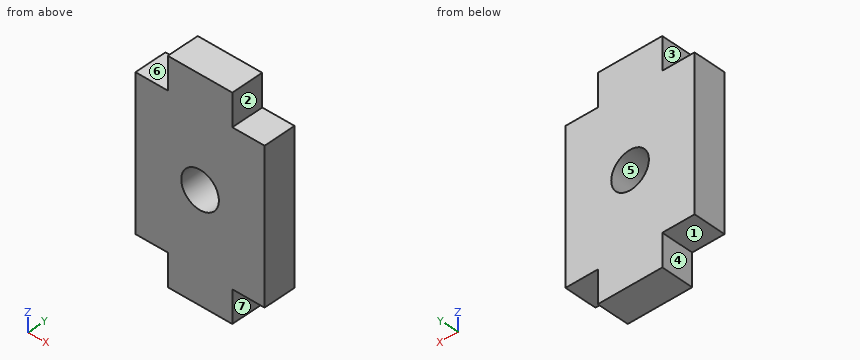
from build123d import *

# Parameters (mm, degrees)
F0_R     = 1.75
F0_W     = 6
F0_H     = 3
F1_DEPTH = 3


with BuildPart() as f1:
    # F0 (on Front) → F1 (new body)
    with BuildSketch(Plane.XZ):
        Polygon((6, -7), (6, 7), (3, 7), (-3, 7), (-6, 7), (-6, -7), (-3, -7), (3, -7), align=None)
        Circle(F0_R, mode=Mode.SUBTRACT)
        with Locations((0, 8.5)):
            Rectangle(F0_W, F0_H)
        with Locations((0, -8.5)):
            Rectangle(F0_W, F0_H)
    extrude(amount=F1_DEPTH)


solid = f1.part
Source: CAD feature listing. Evaluate the final solid. Frame: model axes, mm. Face numbers are marked on the shaded views. A direction names the side the tool comes from. Give positions to 0.01 mm unless a question says otherwise; leave off trailing zeros. Order: outer loops, then holes, each group sorted by start corner. A loop starts at its lowest first (then second) coordinate and runs counter-clockwise, first axis right, second up. Notation, with made-up numbers: (-35.75, 7.5) -> (13.25, 7.5) arc R13 cw to (13.25, 27.5) -> close; hole circle Ø2 at (25.5, 8.5). An arc over 180 degrees is marked (long way). Write item = value, one per line.
Q1. Pin query (flat end, axial travel): pin 1 (0.9 mm diameter, centred on y = -1, z = -8.5, fed in from +X); pin 2 (1.5 mm diameter, centred on x = 4.5, y = -2, fed in from +Z); pin 3 (6 mm diameter, centred on x = -2, z = -1, fed in from +Y); pin 4 (0.9 mm diameter, centred on x = 4, y = -1, fed in from -Z). Return the tip coordinate at first contact, or that it passes through.
Data:
pin_1 = 3
pin_2 = 7
pin_3 = 0
pin_4 = -7
Q2. Set-up query: the marked faces 1, 2 and 3. Return all of +Z, -Z, +X, -X, +Y, -Y with unobstructed straight access to the full face (end or side cutting, diameter ignored); none if empty.
Data:
face_1 = -Z, -X, +Y, -Y
face_2 = +Z, +X, +Y, -Y
face_3 = +Z, -X, +Y, -Y
Q3. Material intervals for line 1 (Z direction, x = 0, y = -1.95); line 2 (Z direction, x = 4.75, y = -1.5); line 3 (X direction, y = -0.55, z = -7.25), sorted ascending. Write a range as from..to.
Data:
line_1 = -10..-1.75, 1.75..10
line_2 = -7..7
line_3 = -3..3
Q4. Pull-direction query (X, two-part tool) for the marked faces 4, 5, 6 and 7; classes: released by +X, released by -X, zero draft, split by the parting line, or undercut.
Data:
face_4 = released by -X
face_5 = undercut
face_6 = zero draft
face_7 = released by +X
Q5. Cut plane D-D, the plane z = 8.75. Output: boundary loops of the cut face in (x, y).
Data:
outline = (-3, -3) -> (3, -3) -> (3, 0) -> (-3, 0) -> close
Q6. Cut plane C-C, the plane y = -1.25. Output: boundary loops of the cut face in (x, z), and give its area (3 significant figures).
Data:
outline = (-6, -7) -> (-3, -7) -> (-3, -10) -> (3, -10) -> (3, -7) -> (6, -7) -> (6, 7) -> (3, 7) -> (3, 10) -> (-3, 10) -> (-3, 7) -> (-6, 7) -> close; hole circle Ø3.5 at (0, 0)
area = 194 mm^2
Q7. Cut plane A-A, the plane z = 0. Output: boundary loops of the cut face in (x, y).
Data:
outline = (-6, -3) -> (-1.75, -3) -> (-1.75, 0) -> (-6, 0) -> close; (1.75, -3) -> (6, -3) -> (6, 0) -> (1.75, 0) -> close
Q8. Cut plane B-B, the plane x = 0. Output: boundary loops of the cut face in (y, z), and give its area (3 significant figures).
Data:
outline = (-3, -10) -> (0, -10) -> (0, -1.75) -> (-3, -1.75) -> close; (-3, 1.75) -> (0, 1.75) -> (0, 10) -> (-3, 10) -> close
area = 49.5 mm^2
